from build123d import *

# Parameters (mm, degrees)
BOSS_EXTRUDE1_DEPTH = 3.175
SKETCH3_R           = 2.413
CUT_EXTRUDE1_DEPTH  = 78.483011202


with BuildPart() as part:
    # Sketch2 → Boss-Extrude1 (new body)
    with BuildSketch(Plane(origin=(0, 0, 0), x_dir=(1, 0, 0), z_dir=(0, 1, 0))):
        Polygon((25.4, 33.02), (50.8, 33.02), (50.8, 58.42), (-25.4, 58.42), (-25.4, 33.02), (0, 33.02), (0, 0), (25.4, 0), align=None)
    extrude(amount=BOSS_EXTRUDE1_DEPTH)

    # Sketch3 → Cut-Extrude1 (cut, through all)
    with BuildSketch(Plane(origin=(0, 3.175, 0), x_dir=(1, 0, 0), z_dir=(0, 1, 0))):
        with Locations(Location((12.7, 13.97, 0), (0, 0, 270))):
            Circle(SKETCH3_R)
        with Locations(Location((-12.7, 45.72, 0), (0, 0, 270))):
            Circle(SKETCH3_R)
        with Locations(Location((12.7, 26.67, 0), (0, 0, 270))):
            Circle(SKETCH3_R)
        with Locations(Location((0, 45.72, 0), (0, 0, 270))):
            Circle(SKETCH3_R)
        with Locations(Location((12.7, 45.72, 0), (0, 0, 270))):
            Circle(SKETCH3_R)
        with Locations(Location((25.4, 45.72, 0), (0, 0, 270))):
            Circle(SKETCH3_R)
        with Locations(Location((38.1, 45.72, 0), (0, 0, 270))):
            Circle(SKETCH3_R)
    extrude(amount=-CUT_EXTRUDE1_DEPTH, mode=Mode.SUBTRACT)


solid = part.part
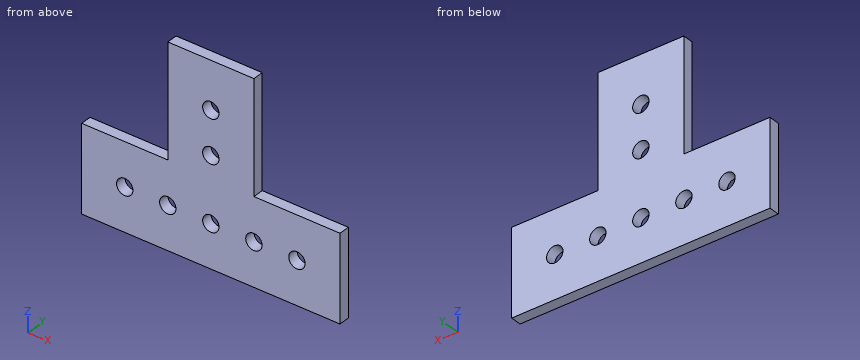
Can you work these out from the model? Positions are in its coordinate system, mm. Coordinates: 2 decimals unless noted, no trailing zeros. Write each loop counter-clockwise with the first axis right and the second up, starting at its lowest first coordinate (ties: lowest second). Pieces come first, ordered by that corner, then holes. Notation, with made-up numbers: (68, 3) -> (122, 3) arc R18 cw to (122, 7) -> close; hole circle Ø3 at (73.5, 76). An arc over 180 degrees is marked (long way). Write each question's results on one line, items separated by ' | '. Start each with the question number.
Q1. I'm going to push flat-ended pins straight in: pin 1 (7.5 mm diameter, centred on x = -12.7, z = -45.72, fed in from -Y); pin 2 (4.5 mm diameter, centred on x = 0, z = -45.72, fed in from -Y); pin 3 (1.5 mm diameter, centred on y = 2.5, z = -25.5, fed in from -X). Where does each tip first touch, or does it pass through?
Q2. If I drill on probe 1 along X at (y, z) = (0.75, -45.72); probe 2 along X at (y, z) = (1.85, -13.97); probe 3 along X at (y, z) = (1.15, -9.5), over which ranges is the centre line in solid material (lowest first)?
Q3. Imagine slicing it at A-A (x = 38.1). Write out the boundary of the cut face in (y, z) (3 decimals), then the cut area to 3 significant figures.
Q4. Imagine slicing it at D-D (x = 12.7). Write out the boundary of the cut face in (y, z) (3 decimals).
Q5. Imagine slicing it at B-B (y = 1.35). Write out the boundary of the cut face in (x, z), then the cut area to 3 significant figures.
Q6. Imagine slicing it at C-C (z = -26.67). Write out the boundary of the cut face in (x, y) (3 decimals).
Taken from the geometry:
1) pin 1: stops at y = 0 | pin 2: passes through | pin 3: stops at x = 0
2) probe 1: x = -25.4 to -15.11, -10.29 to -2.41, 2.41 to 10.29, 15.11 to 22.99, 27.81 to 35.69, 40.51 to 50.8 | probe 2: x = 0 to 10.29, 15.11 to 25.4 | probe 3: x = 0 to 25.4
3) outline: (0, -58.42) -> (3.175, -58.42) -> (3.175, -48.133) -> (0, -48.133) -> close; (0, -43.307) -> (3.175, -43.307) -> (3.175, -33.02) -> (0, -33.02) -> close | area: 65.3 mm^2
4) outline: (0, -58.42) -> (3.175, -58.42) -> (3.175, -48.133) -> (0, -48.133) -> close; (0, -43.307) -> (3.175, -43.307) -> (3.175, -29.083) -> (0, -29.083) -> close; (0, -24.257) -> (3.175, -24.257) -> (3.175, -16.383) -> (0, -16.383) -> close; (0, -11.557) -> (3.175, -11.557) -> (3.175, 0) -> (0, 0) -> close
5) outline: (-25.4, -58.42) -> (50.8, -58.42) -> (50.8, -33.02) -> (25.4, -33.02) -> (25.4, 0) -> (0, 0) -> (0, -33.02) -> (-25.4, -33.02) -> close; hole circle Ø4.83 at (-12.7, -45.72); hole circle Ø4.83 at (0, -45.72); hole circle Ø4.83 at (12.7, -45.72); hole circle Ø4.83 at (12.7, -26.67); hole circle Ø4.83 at (12.7, -13.97); hole circle Ø4.83 at (25.4, -45.72); hole circle Ø4.83 at (38.1, -45.72) | area: 2,650 mm^2
6) outline: (0, 0) -> (10.287, 0) -> (10.287, 3.175) -> (0, 3.175) -> close; (15.113, 0) -> (25.4, 0) -> (25.4, 3.175) -> (15.113, 3.175) -> close
